Check sheet for the modelled part. Datum: model origin and axes. Units: mm. A direction names the side the tool comes from. Coordinates: 2 decimals unless noted, no trailing zeros. Write each loop counter-clockwise with the first axis right and the second up, starting at its lowest first coordinate (ties: lowest second). Pieces come first, ordered by that corner, then holes. Notation, with made-up numbers: M -1,77 L 47,77 A23 cw 47,95 Z; hole C 79,47 d9. An arc over 180 degrees is marked long. Answer as CSV lines item,"result". Start each with the question number.
1) Section check D-D (x = -35). Record the cut outline in (y, z).
2) Go/stop test with flat-tipped pins: pin 1 Ø3 at (x, y) = (-36.5, 4.5) entering from +Z; pin 2 Ø1.8 at (y, z) = (2, -23.5) entering from -X. Record where each tip stops, or that it passes through.
3) Draft check along X on faces 1 (the cylindrical face through (23.289, 2.958, 38.196)), 2 (the cylindrical face through (-42.9, 3, 8)), 3 (the flat face through (15, 3, -27.45)), 4 (the cylindrical face through (-37.548, 2.958, -0.112)). Enter one of: +X half, -X half, draft (parallel to the pull), parting line (faces both ways), or undercut.
4) Material ranges on L1, parallel to Z at x = -17, y = 4.05; L2, parallel to X at y = 4, z = 0; L3, parallel to Z at x = -35, y = 4.75, recorded low to high. Write a range as [from, to].
5) Section check C-C (y = 5.1). State how many separate pieces and enclosed holes the cut face has, and give its area (3 significant figures).
6) Section check A-A (x = -17). Record the cut outline in (y, z), and give its area (3 significant figures).
7) Access from +Z, -Z, +X, -X, +Y, -Y to the whole of each face (thin tool, end or side, straight path). Record for faces 5 (the flat face through (-2, 0, -1)), 6 (the cylindrical face through (18.55, 2.96, -29.94)), 7 (the flat face through (-35, 3, 10)).
8) Section check B-B (z = -30). Record the cut outline in (x, y).
from build123d import *

# Parameters (mm, degrees)
SKETCH_1_R          = 2.55
EXTRUDE_1_DEPTH     = 6
SKETCH_2_R          = 2.55
CUT_EXTRUDE_1_DEPTH = 7


with BuildPart() as part:
    # Эскиз1 → Бобышка-Вытянуть1 (new body)
    with BuildSketch(Plane(origin=(0, 0, 0), x_dir=(1, 0, 0), z_dir=(0, 1, 0))):
        with BuildLine():
            Line((-32, -10), (-38, -10))
            ThreePointArc((-38, -10), (-42.949747468, -7.949747468), (-45, -3))
            Line((-45, -3), (-45, 3))
            ThreePointArc((-45, 3), (-42.949747468, 7.949747468), (-38, 10))
            Line((-38, 10), (-32, 10))
            ThreePointArc((-32, 10), (-27.050252532, 12.050252532), (-25, 17))
            Line((-25, 17), (-25, 34))
            ThreePointArc((-25, 34), (-23.242640687, 38.242640687), (-19, 40))
            Line((-19, 40), (19, 40))
            ThreePointArc((19, 40), (23.242640687, 38.242640687), (25, 34))
            Line((25, 34), (25, -34))
            ThreePointArc((25, -34), (23.242640687, -38.242640687), (19, -40))
            Line((19, -40), (-19, -40))
            ThreePointArc((-19, -40), (-23.242640687, -38.242640687), (-25, -34))
            Line((-25, -34), (-25, -17))
            ThreePointArc((-25, -17), (-27.050252532, -12.050252532), (-32, -10))
        make_face()
        with Locations((-35, 0)):
            Circle(SKETCH_1_R, mode=Mode.SUBTRACT)
        with Locations((18.605, 10)):
            Circle(SKETCH_1_R, mode=Mode.SUBTRACT)
        with Locations((18.605, -10)):
            Circle(SKETCH_1_R, mode=Mode.SUBTRACT)
    extrude(amount=EXTRUDE_1_DEPTH)

    # Эскиз2 → Вырез-Вытянуть1 (cut, through all)
    with BuildSketch(Plane.XZ):
        with Locations((-17, -30)):
            Circle(SKETCH_2_R)
        with Locations((-17, 30)):
            Circle(SKETCH_2_R)
        with BuildLine():
            Line((16, -32.55), (14, -32.55))
            ThreePointArc((14, -32.55), (11.45, -30), (14, -27.45))
            Line((14, -27.45), (16, -27.45))
            ThreePointArc((16, -27.45), (18.55, -30), (16, -32.55))
        make_face()
        with BuildLine():
            Line((16, 32.55), (14, 32.55))
            ThreePointArc((14, 32.55), (11.45, 30), (14, 27.45))
            Line((14, 27.45), (16, 27.45))
            ThreePointArc((16, 27.45), (18.55, 30), (16, 32.55))
        make_face()
    extrude(amount=-CUT_EXTRUDE_1_DEPTH, mode=Mode.SUBTRACT)


solid = part.part
Results found:
1,outline,"M 0,-10 L 6,-10 L 6,-2.55 L 0,-2.55 Z; M 0,2.55 L 6,2.55 L 6,10 L 0,10 Z"
2,pin 1,"stops at z = 10"
2,pin 2,"stops at x = -25"
3,face 1,"+X half"
3,face 2,"-X half"
3,face 3,"undercut"
3,face 4,"undercut"
4,L1,"z = [-40, -32.55], [-27.45, 27.45], [32.55, 40]"
4,L2,"x = [-45, -37.55], [-32.45, 25]"
4,L3,"z = [-10, -2.55], [2.55, 10]"
5,separate pieces,"1"
5,enclosed holes,"7"
5,area,"4,210 mm2"
6,outline,"M 0,-40 L 6,-40 L 6,-32.55 L 0,-32.55 Z; M 0,-27.45 L 6,-27.45 L 6,27.45 L 0,27.45 Z; M 0,32.55 L 6,32.55 L 6,40 L 0,40 Z"
6,area,"419 mm2"
7,face 5,"+Z, -Z, +X, -X, -Y"
7,face 6,"+Y, -Y"
7,face 7,"+Z, -X, +Y, -Y"
8,outline,"M -25,0 L -19.55,0 L -19.55,6 L -25,6 Z; M -14.45,0 L 11.45,0 L 11.45,6 L -14.45,6 Z; M 18.55,0 L 25,0 L 25,6 L 18.55,6 Z"
